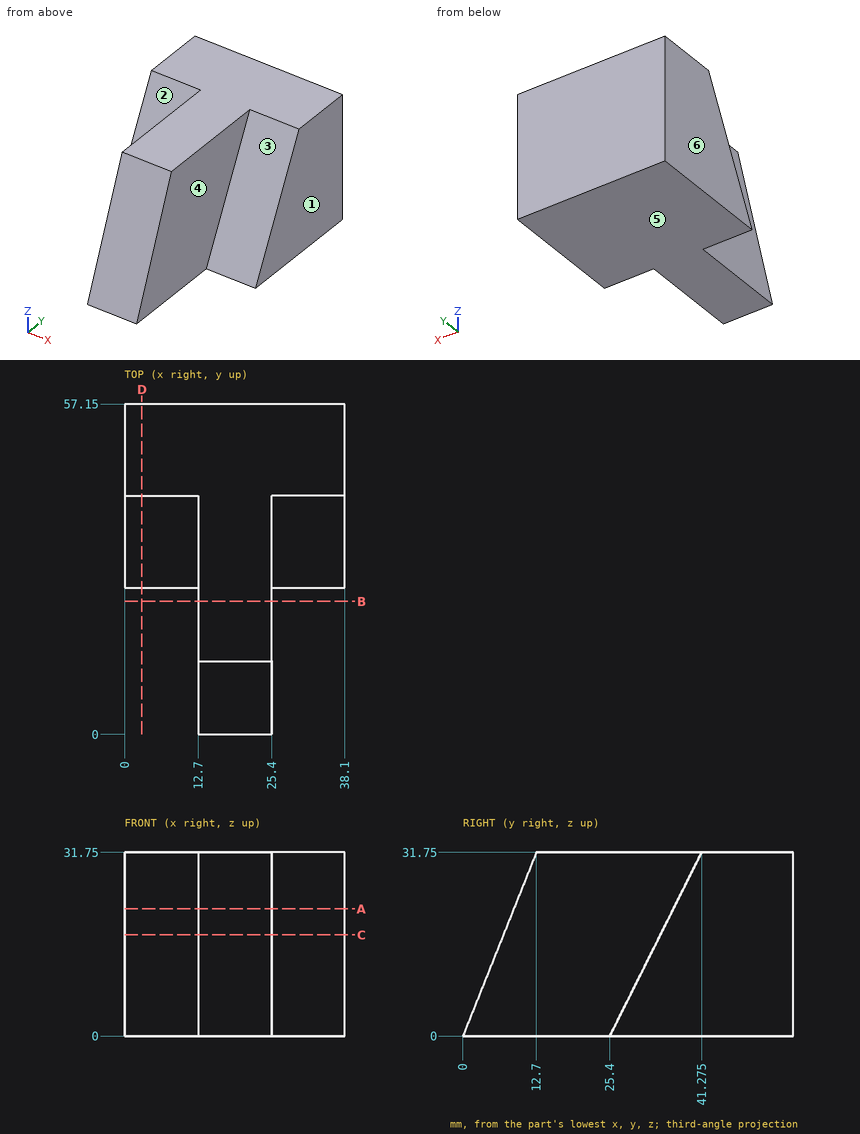
The drawing under review shows one solid part. Ordinate dimensions are in mm from its lowest x, y, z. A direction names the side the tool comes from. Coordinates: 2 decimals unless noted, no trailing zeros. Write each loop counter-clockwise with the first axis right and the second up, starting at its lowest first coordinate (ties: lowest second). Pieces come first, ordered by that corner, then holes. Notation, with made-up numbers: (-21.75, 12.25) - (24.25, 12.25) arc R24 ccw to (24.25, 49.25) - close; hole circle Ø7 at (26, 63.5). An arc over 180 degrees is marked (long way). Put each result on its own line as item: value.
1. Add section A-A, the plane z = 22. Give the boundary of the cut face in (x, y), then the cut area to 3 significant figures.
Values found:
outline: (0, 36.4) - (12.7, 36.4) - (12.7, 8.8) - (25.4, 8.8) - (25.4, 36.4) - (38.1, 36.4) - (38.1, 57.15) - (0, 57.15) - close
area: 1,140 mm²
2. Add section B-B, the plane y = 23. Give the boundary of the cut face in (x, z), then the cut area to 3 significant figures.
Values found:
outline: (12.7, 0) - (25.4, 0) - (25.4, 31.75) - (12.7, 31.75) - close
area: 403 mm²
3. Add section C-C, the plane z = 17.5. Give the boundary of the cut face in (x, y).
Values found:
outline: (0, 34.15) - (12.7, 34.15) - (12.7, 7) - (25.4, 7) - (25.4, 34.15) - (38.1, 34.15) - (38.1, 57.15) - (0, 57.15) - close
4. Wall thickness on probe 1 along X at (y, z) = (33, 25); probe 2 along Y at (x, z) = (31, 7); probe 3 along Y at (x, z) = (17.5, 11): over which ranges is each line inside the solid? List them lowest first.
Values found:
probe 1: 12.7 to 25.4
probe 2: 28.9 to 57.15
probe 3: 4.4 to 57.15
5. For pin 1 (1 mm diameter, centred on y = 21.5, z = 10, fed in from -X); pin 2 (1 mm diameter, centred on y = 11, z = 12.5, fed in from +X), all flat-tipped, find the tip position at first contact; note any pin that passes through.
Values found:
pin 1: x = 12.7
pin 2: x = 25.4
6. Mouldability with a two-part tool opening along X and no side actions: class the marked faces 4, 5 and 6 as released by +X, released by -X, zero draft, split by the parting line, or undercut.
Values found:
face 4: released by +X
face 5: zero draft
face 6: released by -X
7. Machinability: for the marked faces 1, 2 and 3, which of the approach directions +Z, -Z, +X, -X, +Y, -Y give a long, thin tool a straight path to every point of the face, cutting with its end or side? Answer none if there is none.
Values found:
face 1: +Z, -Z, +X, +Y, -Y
face 2: +Z, -X, -Y
face 3: +Z, +X, -Y
8. Add section D-D, the plane x = 3. Give the boundary of the cut face in (y, z) (3 decimals).
Values found:
outline: (25.4, 0) - (57.15, 0) - (57.15, 31.75) - (41.275, 31.75) - close
